from build123d import *

# Parameters (mm, degrees)
SKETCH_1_R      = 12
SKETCH_1_R_2    = 2
EXTRUDE_1_DEPTH = 4
CHAMFER_1_SIZE  = 0.5


with BuildPart() as part:
    # 草图1 → 凸台-拉伸1 (new body)
    with BuildSketch(Plane.XY):
        Circle(SKETCH_1_R)
        with Locations((0, 5)):
            Circle(SKETCH_1_R_2, mode=Mode.SUBTRACT)
        with Locations((4.330127019, -2.5)):
            Circle(SKETCH_1_R_2, mode=Mode.SUBTRACT)
        with Locations((-4.330127019, -2.5)):
            Circle(SKETCH_1_R_2, mode=Mode.SUBTRACT)
    extrude(amount=EXTRUDE_1_DEPTH)

    # 倒角1
    chamfer_1_edges = [part.edges().sort_by_distance(p)[0] for p in [
        (-12, 0, 0),
        (-12, 0, 4),
    ]]
    chamfer(chamfer_1_edges, length=CHAMFER_1_SIZE)


solid = part.part
Read the model definition and answer for the solid it produces. Units are mm, in the model's axes. Give positions to 0.01 mm unless a question says otherwise; leave off trailing zeros. Write each loop counter-clockwise with the first axis right and the second up, starting at its lowest first coordinate (ties: lowest second). Pieces come first, ordered by that corner, then holes. Notation, with made-up numbers: (84.5, 45.5) -> (143.5, 45.5) arc R20 ccw to (143.5, 57.5) -> close; hole circle Ø11 at (78.5, 42.5). An arc over 180 degrees is marked (long way). Answer as a JSON object with one key per item and string values. Group by question number.
1) This flat-tipped pin is pushed along its axis until it touches: P1, Ø1.5, axis at y = -4.5, z = 2, coming from the +X side. Where does it stop, or does it pass through?
2) Find section C-C (y = -2.5). Count the separate pieces of the cut face and the enclosed holes in it, and give its area (3 significant figures).
3) Find section A-A (x = 0). Write down the section's boundary in (y, z), and give its area (3 significant figures).
4) Find section B-B (z = 2.6). Write down the section's boundary in (x, y).
5) Consider L1, parallel to Y at x = 0, z = 2; L2, parallel to X at y = -4, z = 2.4; L3, parallel to X at y = -0.75, z = 3.65. Determine where each line is inside the solid, lowest interval first. Write a range as from..to.
6) The mould has two halves that part along X. Classify faces 1 (the cylindrical face through (-5.917, -3.717, 1.972)), 2 (the flat face through (0, 0, 4)), 3 (the cylindrical face through (-11.99, 0.53, 1.98)): +X half, -X half, draft (parallel to the pull), parting line (faces both ways), or undercut.
Values follow:
{
 "1": {"P1": "stops at x = 11.4"},
 "2": {"separate pieces": "3", "enclosed holes": "0", "area": "61.4 mm2"},
 "3": {"outline": "(-12, 0.5) -> (-11.5, 0) -> (3, 0) -> (3, 4) -> (-11.5, 4) -> (-12, 3.5) -> close; (7, 0) -> (11.5, 0) -> (12, 0.5) -> (12, 3.5) -> (11.5, 4) -> (7, 4) -> close", "area": "79.5 mm2"},
 "4": {"outline": "circle Ø24 at (0, 0); hole circle Ø4 at (-4.33, -2.5); hole circle Ø4 at (0, 5); hole circle Ø4 at (4.33, -2.5)"},
 "5": {"L1": "y = -12..3, 7..12", "L2": "x = -11.31..-5.65, -3.01..3.01, 5.65..11.31", "L3": "x = -11.83..-5.3, -3.36..3.36, 5.3..11.83"},
 "6": {"face 1": "undercut", "face 2": "draft", "face 3": "parting line"}
}
